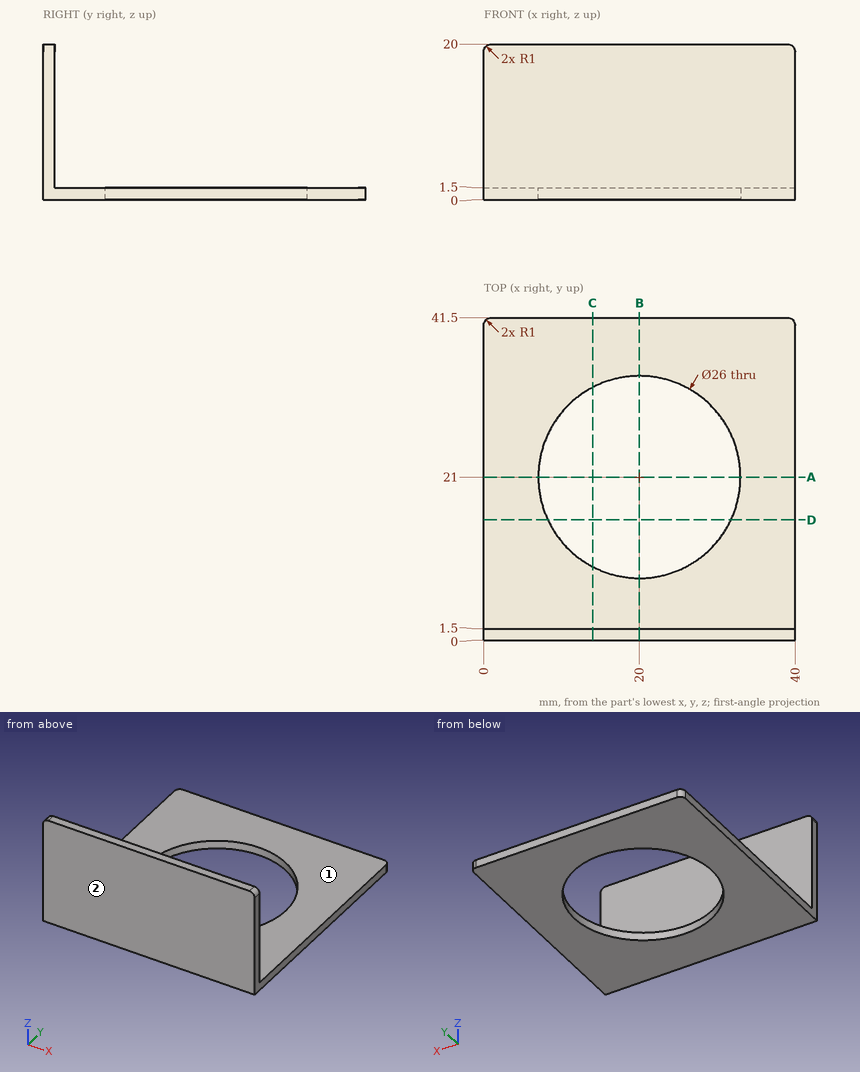
Geometry check sheet. Reference: drawing and pictorial views, mm from the part's lowest x, y, z. A direction names the side the tool comes from. Round coordinates to 2 decimals unless told otherwise and drop trailing zeros. Order: outer loops, then holes, each group sorted by start corner. A loop starts at its lowest first (then second) coordinate and runs counter-clockwise, first axis right, second up. Notation, with made-up numbers: (25, -25) - (61, -25) arc R24 ccw to (61, -2) - close; hole circle Ø7 at (4.5, 60.5). An arc over 180 degrees is marked (long way). One line per question, with ' | ' between items. Start each with the question number.
(1) Sectioned sample at C-C on x = 14. Record the cut outline in (y, z), and give its area (3 significant figures).
(2) Sectioned sample at A-A on y = 21. Record the cut outline in (x, z).
(3) Sectioned sample at B-B on x = 20. Record the cut outline in (y, z), and give its area (3 significant figures).
(4) Sectioned sample at D-D on y = 15.5. Record the cut outline in (x, z), and give its area (3 significant figures).
(5) Access from +Z, -Z, +X, -X, +Y, -Y to the whole of each face (thin tool, end or side, straight path). Record for the marked faces 1 and 2.
(6) Depth check by flat-ended pin: pin 1 Ø3 at (x, y) = (6.5, 32) entering from +Z; pin 2 Ø5.5 at (x, z) = (25, 13.5) entering from +Y. Enter the tip coordinate at first touch or a pass-through.
(7) Thickness scan on L1, parallel to Y at x = 20, z = 0.75; L2, parallel to Z at x = 15, y = 36.5. Record the ranges inside material, lowest first. Write a range as [from, to].
Conclusion:
1) outline: (0, 0) - (9.47, 0) - (9.47, 1.5) - (1.5, 1.5) - (1.5, 20) - (0, 20) - close; (32.53, 0) - (41.5, 0) - (41.5, 1.5) - (32.53, 1.5) - close | area: 55.4 mm2
2) outline: (0, 0) - (7, 0) - (7, 1.5) - (0, 1.5) - close; (33, 0) - (40, 0) - (40, 1.5) - (33, 1.5) - close
3) outline: (0, 0) - (8, 0) - (8, 1.5) - (1.5, 1.5) - (1.5, 20) - (0, 20) - close; (34, 0) - (41.5, 0) - (41.5, 1.5) - (34, 1.5) - close | area: 51.0 mm2
4) outline: (0, 0) - (8.22, 0) - (8.22, 1.5) - (0, 1.5) - close; (31.78, 0) - (40, 0) - (40, 1.5) - (31.78, 1.5) - close | area: 24.7 mm2
5) face 1: +Z, +X, -X, +Y | face 2: +Z, -Z, +X, -X, -Y
6) pin 1: stops at z = 1.5 | pin 2: stops at y = 1.5
7) L1: y = [0, 8], [34, 41.5] | L2: z = [0, 1.5]
